For this review, take the finished solid that the model builds, in its own axes (mm). A direction names the side the tool comes from. Give positions to 0.01 mm unless a question says otherwise; leave off trailing zeros. Write each loop counter-clockwise with the first axis right and the second up, starting at its lowest first coordinate (ties: lowest second). Pieces come first, ordered by that corner, then holes. Notation, with made-up numbers: (-8, -13.5) -> (41, -13.5) arc R6 cw to (41, -3.5) -> close; hole circle Ø4 at (67, 76.5). An arc over 180 degrees is marked (long way). Return JSON: item names as keys, results as strings.
from build123d import *

# Parameters (mm, degrees)
F0_W          = 16
F0_H          = 13.5
F1_DEPTH      = 13.5
F2_R          = 4.75
F3_DEPTH      = 11.5
F4_R          = 5.5
F5_DEPTH      = 2
F7_DEPTH      = 11
F8_R          = 3.05
F9_DEPTH      = 17
F10_W         = 9.2
F10_H         = 2.4967868254
F11_DEPTH     = 10
F12_W         = 12.1366479748
F12_H         = 1.7
F13_DEPTH     = 8
F14_T4_DEPTH  = 19.347977845
F14_T9_DEPTH  = 19.347977845
F14_T11_DEPTH = 31
F15_R         = 1.5
F16_SIZE      = 0.1


# Not quite as in the source:
# - a fillet or chamfer that OpenCascade refuses, or shapes differently, is made with other operations: its cross-section is extruded or revolved along the edge and cut away or added


with BuildPart() as f1:
    # F0 (on Top) → F1 (new body)
    with BuildSketch(Plane.XY):
        Rectangle(F0_W, F0_H)
    extrude(amount=F1_DEPTH)

    # F2 (on face) → F3 (join)
    with BuildSketch(Plane.YZ.offset(8)):
        with Locations((0, 6.75)):
            Circle(F2_R)
    extrude(amount=F3_DEPTH)

    # F4 (on face) → F5 (join)
    with BuildSketch(Plane.YZ.offset(19.5)):
        with Locations((0, 6.75)):
            Circle(F4_R)
    extrude(amount=F5_DEPTH)

    # F6 (on face) → F7 (cut)
    with BuildSketch(Plane.XY.offset(13.5)):
        Polygon((0, 3.3), (0, 1.8), (-8, 4.6), (-8, -4.6), (0, -1.8), (0, -3.3), (-4.5499948867, -4.6), (3.847977845, -4.6), (4.6067554504, -3.4655697951), (6, -3.4655697951), (6, 4.0877170554), (4.6067554504, 4.0877170554), (3.847977845, 4.6), (-4.5499948867, 4.6), align=None)
    extrude(amount=-F7_DEPTH, mode=Mode.SUBTRACT)

    # F8 (on face) → F9 (cut)
    with BuildSketch(Plane.YZ.offset(21.5)):
        with Locations((0, 6.75)):
            Circle(F8_R)
    extrude(amount=-F9_DEPTH, mode=Mode.SUBTRACT)

    # F10 (on face) → F11 (cut)
    with BuildSketch(Plane(origin=(-8, 0, 0), x_dir=(0, -1, 0), z_dir=(-1, 0, 0))):
        with Locations((0, 3.7483934127)):
            Rectangle(F10_W, F10_H)
    extrude(amount=-F11_DEPTH, mode=Mode.SUBTRACT)

    # F12 (on face) → F13 (cut)
    with BuildSketch(Plane.YZ.offset(21.5)):
        with Locations((0, 6.75)):
            Rectangle(F12_W, F12_H)
    extrude(amount=-F13_DEPTH, mode=Mode.SUBTRACT)

    # F14: fillet of radius 3 on 4 edges, made by hand


with BuildPart() as f14_tool2:
    # F14_s3 → F14_t4 (new body)
    with BuildSketch(Plane.YZ.offset(11.347977845)):
        with BuildLine():
            ThreePointArc((1.6, 2.5), (3.7213203436, 3.3786796564), (4.6, 5.5))
            Line((4.6, 5.5), (4.6, 2.5))
            Line((4.6, 2.5), (1.6, 2.5))
        make_face()
    extrude(amount=-F14_T4_DEPTH)

    split(bisect_by=Plane.YZ.offset(6), keep=Keep.BOTTOM)


with BuildPart() as f1_1:
    add(f1.part)

    # F14_t1: union F14_tool2
    add(f14_tool2.part)


with BuildPart() as f14_tool7:
    # F14_s8 → F14_t9 (new body)
    with BuildSketch(Plane.YZ.offset(-8)):
        with BuildLine():
            ThreePointArc((-1.6, 2.5), (-3.7213203436, 3.3786796564), (-4.6, 5.5))
            Line((-4.6, 5.5), (-4.6, 2.5))
            Line((-4.6, 2.5), (-1.6, 2.5))
        make_face()
    extrude(amount=F14_T9_DEPTH)

    split(bisect_by=Plane.YZ.offset(6), keep=Keep.BOTTOM)


with BuildPart() as f1_2:
    add(f1_1.part)

    # F14_t6: union F14_tool7
    add(f14_tool7.part)

    # F14_s12 → F14_t11 (cut)
    with BuildSketch(Plane.YZ.offset(-15.5)):
        with BuildLine():
            ThreePointArc((3.75, 0), (5.8713203436, 0.8786796564), (6.75, 3))
            Line((6.75, 3), (6.75, 0))
            Line((6.75, 0), (3.75, 0))
        make_face()
        with BuildLine():
            ThreePointArc((-6.75, 3), (-5.8713203436, 0.8786796564), (-3.75, 0))
            Line((-3.75, 0), (-6.75, 0))
            Line((-6.75, 0), (-6.75, 3))
        make_face()
    extrude(amount=F14_T11_DEPTH, mode=Mode.SUBTRACT)

    # F15
    f15_edges = [f1_2.edges().sort_by_distance(p)[0] for p in [
        (21.5, 0, 12.25),
        (21.5, 0, 1.25),
    ]]
    fillet(f15_edges, radius=F15_R)

    # F16
    f16_edges = [f1_2.edges().sort_by_distance(p)[0] for p in [
        (19.5, 0, 1.25),
        (19.5, 0, 12.25),
    ]]
    chamfer(f16_edges, length=F16_SIZE)


solid = f1_2.part
1. The part is to be moulded in two halves that separate along Y. For faces 1 (the flat face through (0, -6.75, 8)), 2 (the flat face through (-8, 0, 2)), 3 (the cylindrical face through (-1.1, -3.7, 3.36)), say which applies: +Y half, -Y half, draft (parallel to the pull), parting line (faces both ways), or undercut.
Results found:
{"face 1": "-Y half", "face 2": "draft", "face 3": "undercut"}
2. Add section A-A, the plane z = 6.75. State the section outline as (x, y) points.
Results found:
{"outline": "(-8, -6.75) -> (8, -6.75) -> (8, -4.75) -> (13.5, -4.75) -> (13.5, -3.05) -> (6, -3.05) -> (6, -3.47) -> (4.61, -3.47) -> (3.85, -4.6) -> (-4.55, -4.6) -> (0, -3.3) -> (0, -1.8) -> (-8, -4.6) -> close; (-8, 4.6) -> (0, 1.8) -> (0, 3.3) -> (-4.55, 4.6) -> (3.85, 4.6) -> (4.61, 4.09) -> (6, 4.09) -> (6, 3.05) -> (13.5, 3.05) -> (13.5, 4.75) -> (8, 4.75) -> (8, 6.75) -> (-8, 6.75) -> close"}
3. Add section C-C, the plane x = -1.75. State the section outline as (y, z) points, plus the area to 3 significant figures.
Results found:
{"outline": "(-6.75, 3) arc R3 ccw to (-3.75, 0) -> (3.75, 0) arc R3 ccw to (6.75, 3) -> (6.75, 13.5) -> (4.6, 13.5) -> (4.6, 5.5) arc R3 cw to (1.6, 2.5) -> (-1.6, 2.5) arc R3 cw to (-4.6, 5.5) -> (-4.6, 13.5) -> (-6.75, 13.5) -> close; (-3.8, 5) -> (-2.41, 5) -> (-2.41, 13.5) -> (-3.8, 13.5) -> close; (2.41, 5) -> (3.8, 5) -> (3.8, 13.5) -> (2.41, 13.5) -> close", "area": "105 mm²"}
4. To check wall thickness, follow probe 1 along Z at (x, y) = (16.25, 0); probe 2 along Y at (x, z) = (12.75, 6.75); probe 3 along Y at (x, z) = (1.75, 12.75). State the ranges of each line that lie inside material, in increasing order.
Results found:
{"probe 1": "z = 2 to 3.7, 9.8 to 11.5", "probe 2": "y = -4.75 to -3.05, 3.05 to 4.75", "probe 3": "y = -6.75 to -4.6, 4.6 to 6.75"}
5. For faces 4 (the cylindrical face through (19.8, 0.11, 12.25)), 5 (the flat face through (18, -4, 5.9)), 6 (the flat face through (0, 3, 9)), list the 3-axis set-ups (+Z, -Z, +X, -X, +Y, -Y) from which the entire face can be reached by the end or side of a thin tool; tool diameter is ignored.
Results found:
{"face 4": "+Z, +X", "face 5": "+X, +Y, -Y", "face 6": "+Z"}
6. Add section D-D, the plane x = 2. State the section outline as (y, z) points.
Results found:
{"outline": "(-6.75, 3) arc R3 ccw to (-3.75, 0) -> (3.75, 0) arc R3 ccw to (6.75, 3) -> (6.75, 13.5) -> (4.6, 13.5) -> (4.6, 5.5) arc R3 cw to (1.6, 2.5) -> (-1.6, 2.5) arc R3 cw to (-4.6, 5.5) -> (-4.6, 13.5) -> (-6.75, 13.5) -> close"}
7. Add section B-B, the plane y = 0. State the section outline as (x, z) points, plus the area to 3 significant figures.
Results found:
{"outline": "(-8, 0) -> (8, 0) -> (8, 2) -> (19.5, 2) -> (19.5, 1.35) -> (19.6, 1.25) -> (20, 1.25) arc R1.5 ccw to (21.5, 2.75) -> (21.5, 3.7) -> (6, 3.7) -> (6, 2.5) -> (-8, 2.5) -> close; (6, 9.8) -> (21.5, 9.8) -> (21.5, 10.75) arc R1.5 ccw to (20, 12.25) -> (19.6, 12.25) -> (19.5, 12.15) -> (19.5, 11.5) -> (8, 11.5) -> (8, 13.5) -> (6, 13.5) -> close", "area": "97.7 mm²"}
8. For pin 1 (3 mm diameter, centred on x = 17.5, y = 4, fed in from +Z); pin 2 (1.3 mm diameter, centred on x = 17, y = 4.5, fed in from -Z); pin 3 (3 mm diameter, centred on x = 17.5, y = -4.5, fed in from -Z); pin 4 (3.5 mm diameter, centred on y = 1.5, z = 4, fed in from -X), all flat-tipped, find the tip position at first contact; note any pin that passes through.
Results found:
{"pin 1": "stops at z = 10.79", "pin 2": "stops at z = 3.97", "pin 3": "stops at z = 3.07", "pin 4": "stops at x = -8"}
